Source: CAD feature listing. Evaluate the final solid. Frame: model axes, mm. Give positions to 0.01 mm unless a question says otherwise; leave off trailing zeros. Loops run counter-clockwise (first coordinate to the right, second up) from the corner with the lowest first, then second, coordinate; pieces in that order, holes last. Notation, with made-up numbers: M 68,25.5 L 82,25.5 A5 cw 82,32.5 Z; hole C -24,0 d3. An arc over 180 degrees is marked long. Answer in a Markdown table with one row per item.
```python
from build123d import *

# Parameters (mm, degrees)
SKETCH1_R           = 8
SKETCH1_R_2         = 6
SKETCH1_R_3         = 2.5
SKETCH1_W           = 72
SKETCH1_H           = 26
SKETCH1_W_2         = 36
SKETCH1_H_2         = 50
BOSS_EXTRUDE1_DEPTH = 5


with BuildPart() as part:
    # Sketch1 → Boss-Extrude1 (new body)
    with BuildSketch(Plane.XY):
        with BuildLine():
            Line((140, -92.5), (-140, -92.5))
            ThreePointArc((-140, -92.5), (-147.071067812, -89.571067812), (-150, -82.5))
            Line((-150, -82.5), (-150, 42.5))
            ThreePointArc((-150, 42.5), (-135.355339059, 77.855339059), (-100, 92.5))
            Line((-100, 92.5), (100, 92.5))
            ThreePointArc((100, 92.5), (135.355339059, 77.855339059), (150, 42.5))
            Line((150, 42.5), (150, -82.5))
            ThreePointArc((150, -82.5), (147.071067812, -89.571067812), (140, -92.5))
        make_face()
        with Locations((-13, -72.5)):
            Circle(SKETCH1_R, mode=Mode.SUBTRACT)
        with Locations(Location((13, -72.5, 0), (0, 0, 180))):
            Circle(SKETCH1_R, mode=Mode.SUBTRACT)
        with Locations((100, 17.5)):
            Circle(SKETCH1_R_2, mode=Mode.SUBTRACT)
        with Locations((-120, 17.5)):
            Circle(SKETCH1_R_3, mode=Mode.SUBTRACT)
        with Locations((-100, 17.5)):
            Circle(SKETCH1_R_3, mode=Mode.SUBTRACT)
        with Locations((-80, 17.5)):
            Circle(SKETCH1_R_3, mode=Mode.SUBTRACT)
        with Locations((-98, -22.5)):
            Rectangle(SKETCH1_W, SKETCH1_H, mode=Mode.SUBTRACT)
        with Locations((0, 47.5)):
            Rectangle(SKETCH1_W, SKETCH1_H, mode=Mode.SUBTRACT)
        with Locations((98, -22.5)):
            Rectangle(SKETCH1_W, SKETCH1_H, mode=Mode.SUBTRACT)
        with Locations((0, -22.5)):
            Rectangle(SKETCH1_W_2, SKETCH1_H_2, mode=Mode.SUBTRACT)
    extrude(amount=BOSS_EXTRUDE1_DEPTH)


solid = part.part
```
1) Material intervals for L1, parallel to X at y = -24.5, z = 2.4; L2, parallel to Y at x = -80, z = 3.9; L3, parallel to Y at x = 100, z = 2.8, sorted ascending.
Reply:
| item | result |
|---|---|
| L1 | x = -150 to -134, -62 to -18, 18 to 62, 134 to 150 |
| L2 | y = -92.5 to -35.5, -9.5 to 15, 20 to 92.5 |
| L3 | y = -92.5 to -35.5, -9.5 to 11.5, 23.5 to 92.5 |
2) Section C-C, the plane x = -13. Return loops of the section in (y, z).
Reply:
| item | result |
|---|---|
| outline | M -92.5,0 L -80.5,0 L -80.5,5 L -92.5,5 Z; M -64.5,0 L -47.5,0 L -47.5,5 L -64.5,5 Z; M 2.5,0 L 34.5,0 L 34.5,5 L 2.5,5 Z; M 60.5,0 L 92.5,0 L 92.5,5 L 60.5,5 Z |
3) Section B-B, the plane z = 3.15. Count the separate pieces of the cut face and the enclosed holes in it, then the cut area to 3 significant figures.
Reply:
| item | result |
|---|---|
| separate pieces | 1 |
| enclosed holes | 10 |
| area | 46,400 mm² |
4) Pin query (flat end, axial travel): pin 1 Ø2.5 at (x, z) = (-108.5, 2.5) entering from +Y; pin 2 Ø6 at (x, y) = (3, 33) entering from -Z. Return the tip coordinate at first contact, or that it passes through.
Reply:
| item | result |
|---|---|
| pin 1 | stops at y = 91.97 |
| pin 2 | stops at z = 0 |
5) Section A-A, the plane y = -72.5. Return loops of the section in (x, z).
Reply:
| item | result |
|---|---|
| outline | M -150,0 L -21,0 L -21,5 L -150,5 Z; M -5,0 L 5,0 L 5,5 L -5,5 Z; M 21,0 L 150,0 L 150,5 L 21,5 Z |
6) Pull-direction query (Y, two-part tool) for faces 1 (the cylindrical face through (14.041, -80.432, 2.465)), 2 (the flat face through (2, 22, 0)), 3 (the cylindrical face through (-146.99, -89.65, 2.46)); classes: released by +Y, released by -Y, zero draft, split by the parting line, or undercut.
Reply:
| item | result |
|---|---|
| face 1 | undercut |
| face 2 | zero draft |
| face 3 | released by -Y |
7) Section D-D, the plane x = -108. Return loops of the section in (y, z).
Reply:
| item | result |
|---|---|
| outline | M -92.5,0 L -35.5,0 L -35.5,5 L -92.5,5 Z; M -9.5,0 L 91.86,0 L 91.86,5 L -9.5,5 Z |
